Could you check a few things on this drawing? It's one solid part, dimensions in mm from its lowest x, y, z. Coordinates: 2 decimals unless noted, no trailing zeros. Write each loop counter-clockwise with the first axis right and the second up, starting at its lowest first coordinate (ties: lowest second). Pieces come first, ordered by that corner, then holes. Notation, with made-up numbers: (50, -39) - (90, -39) arc R8 ccw to (90, -30) - close; hole circle Ø7 at (-27.5, 40.5). An arc over 180 degrees is marked (long way). Answer as a JSON object with one key per item and string values. Group by question number.
1) Will these pins go through, and if not, where does the flat tip stop? pin 1 Ø1.3 at (x, y) = (41, 2) entering from +Z; pin 2 Ø1.3 at (x, y) = (96.5, 1.5) entering from -Z; pin 3 Ø1 at (y, z) = (0.5, 22) entering from -X.
2) Please list where this line runs through material, in increasing order: line 1 along Z through (x, y) = (50.5, 1.95).
3) If we section it at A-A (x = 19): Write out the boundary of the cut face in (y, z).
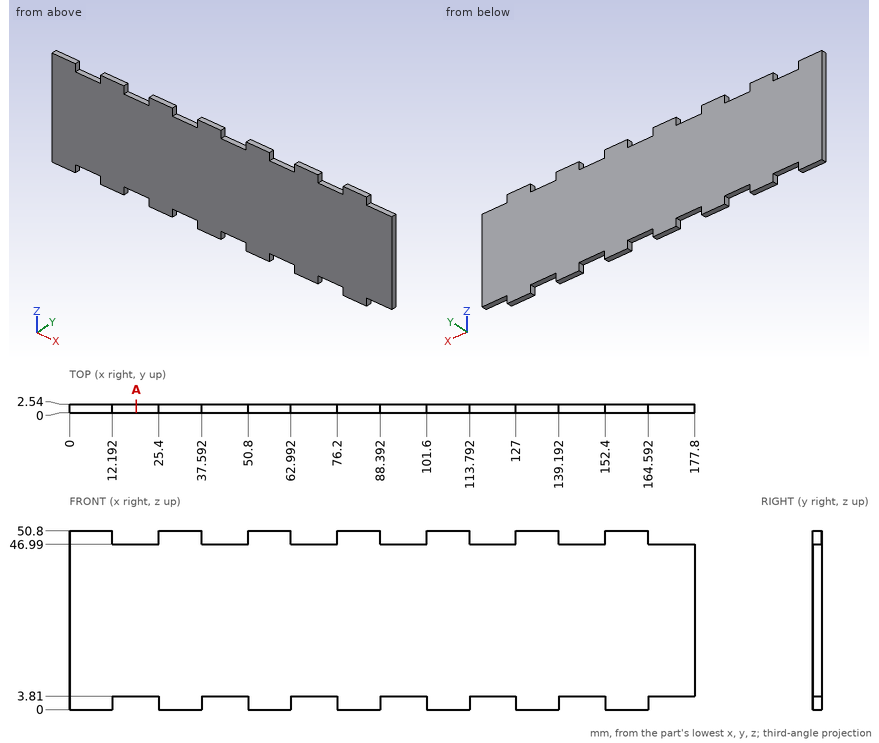
Here are the results:
{
 "1": {"pin 1": "stops at z = 46.99", "pin 2": "stops at z = 3.81", "pin 3": "stops at x = 0"},
 "2": {"line 1": "z = 3.81 to 46.99"},
 "3": {"outline": "(0, 3.81) - (2.54, 3.81) - (2.54, 46.99) - (0, 46.99) - close"}
}
